The figure shows three views and two pictorial views of one solid part (mm, origin at its lowest corner). Answer the questions. A direction names the side the tool comes from. Coordinates: 2 decimals unless noted, no trailing zeros. Loops run counter-clockwise (first coordinate to the right, second up) from the corner with the lowest first, then second, coordinate; pieces in that order, holes last. Notation, with made-up numbers: M 61.25,78 L 97.25,78 A22 ccw 97.25,115 Z; hole C 58.5,45.5 d5. An arc over 180 degrees is marked long. Answer as a JSON object with one key per item and string values. Group by question number.
1. Determine the mould class of the marked faces 3, 4 and 5 for opening direction Z: released by +Z, released by -Z, zero draft, split by the parting line, or undercut.
2. A cutting plane is placed at C-C on y = 7. Give the vertices of the cut face in (x, z).
3. A cutting plane is placed at D-D on x = 165.1. Give the vertices of the cut face in (y, z).
4. A cutting plane is placed at A-A on z = 25.4. Give the vertices of the cut face in (x, y).
5. For the marked faces 1 and 2, determine the directions among +Z, -Z, +X, -X, +Y, -Y from which every point of the face is accessible in a straight line to the end or side of a thin tool.
6. A cutting plane is placed at B-B on x = 109. Give the vertices of the cut face in (y, z).
7. Straight lines are drawn through the part: L1, parallel to Z at x = 177.8, y = 24.5; L2, parallel to Y at x = 132, z = 4.5; L3, parallel to Z at x = 60, y = 7.75. For each, find the intervals that lie inside material, in ascending order.
8. Given pin 1 (4 mm diameter, centred on x = 203.2, z = 38.1, fed in from -Y); pin 2 (6.5 mm diameter, centred on x = 165.1, y = 12.7, fed in from +Z), each flat-ended and moving along its own axis, determine where each tip first touches the part or whether it passes through.
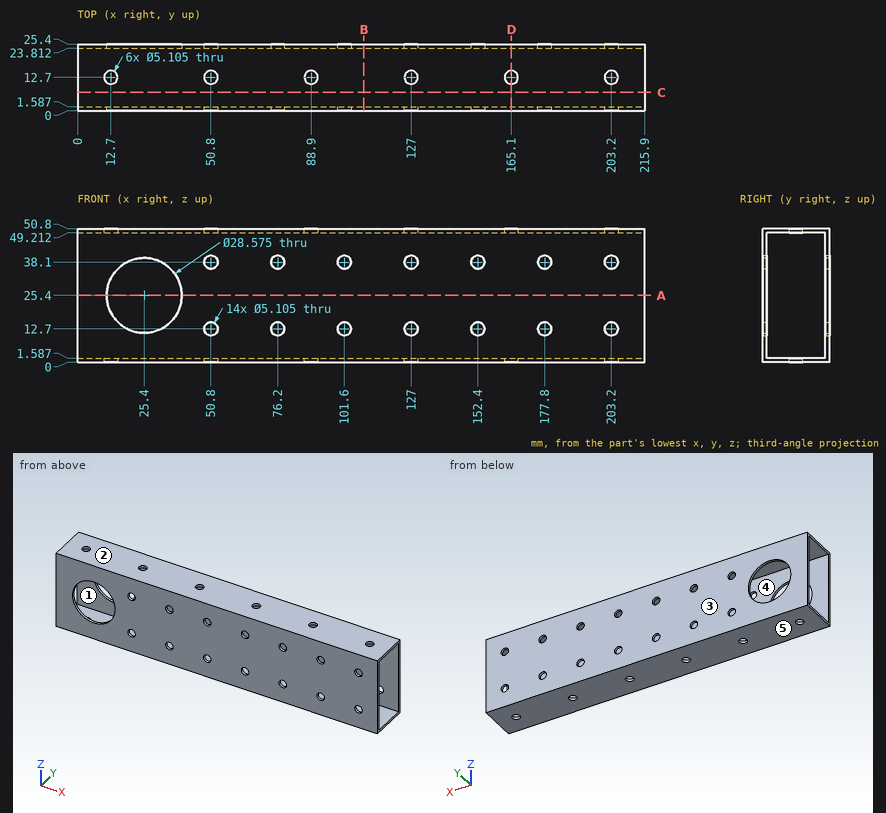
From the geometry:
{
 "1": {"face 3": "zero draft", "face 4": "undercut", "face 5": "released by -Z"},
 "2": {"outline": "M 0,0 L 215.9,0 L 215.9,1.59 L 0,1.59 Z; M 0,49.21 L 215.9,49.21 L 215.9,50.8 L 0,50.8 Z"},
 "3": {"outline": "M 0,0 L 10.15,0 L 10.15,1.59 L 1.59,1.59 L 1.59,49.21 L 10.15,49.21 L 10.15,50.8 L 0,50.8 Z; M 15.25,0 L 25.4,0 L 25.4,50.8 L 15.25,50.8 L 15.25,49.21 L 23.81,49.21 L 23.81,1.59 L 15.25,1.59 Z"},
 "4": {"outline": "M 0,0 L 11.11,0 L 11.11,1.59 L 0,1.59 Z; M 0,23.81 L 11.11,23.81 L 11.11,25.4 L 0,25.4 Z; M 39.69,0 L 215.9,0 L 215.9,1.59 L 39.69,1.59 Z; M 39.69,23.81 L 215.9,23.81 L 215.9,25.4 L 39.69,25.4 Z"},
 "5": {"face 1": "+X, -X", "face 2": "+Z, +X, -X, +Y, -Y"},
 "6": {"outline": "M 0,0 L 25.4,0 L 25.4,50.8 L 0,50.8 Z; hole M 1.59,1.59 L 23.81,1.59 L 23.81,49.21 L 1.59,49.21 Z"},
 "7": {"L1": "z = 0 to 10.15, 15.25 to 35.55, 40.65 to 50.8", "L2": "y = 0 to 1.59, 23.81 to 25.4", "L3": "z = 0 to 1.59, 49.21 to 50.8"},
 "8": {"pin 1": "passes through", "pin 2": "stops at z = 50.8"}
}
